Read the model definition and answer for the solid it produces. Units are mm, in the model's axes. Face numbers are marked on the shaded views. A direction names the side the tool comes from. Round coordinates to 2 decimals unless told otherwise and drop trailing zeros. Order: outer loops, then holes, each group sorted by start corner. A loop starts at its lowest first (then second) coordinate and runs counter-clockwise, first axis right, second up. Notation, with made-up numbers: (72, 40) - (84, 40) arc R17 ccw to (84, 70) - close; hole circle Ø10 at (37, -31). An arc over 180 degrees is marked (long way). Put each result on its own line as item: value. Start each with the question number.
Q1. Section D-D on y = -120 is taken. Give the vertices of the cut face in (x, z).
Q2. Section C-C on z = 0 is taken. Give the vertices of the cut face in (x, y).
Q3. Which of the six approach directions +Z, -Z, +X, -X, +Y, -Y give full straight-line access (tool end or side, diameter ignored) to the marked faces 5, 6 and 7?
Q4. Find the intervals of material crossed by line 1 along Y through (x, z) = (0, -2.25); line 2 along Y through (x, z) = (3.5, -7.25); line 3 along Y through (x, z) = (-1, 1.5), in increasing order. Write a range as from..to.
Q5. Each of these flat-tipped pins is pushed along its axis until it touches: pin 1 Ø2 at (x, y) = (10, -40) entering from -Z; pin 2 Ø12 at (x, y) = (-3, -66.5) entering from +Z; pin 3 Ø6 at (y, z) = (-37.5, 0.5) entering from -X; pin 4 Ø5.5 at (x, y) = (2.5, 21) entering from +Z. Where does it stop, or does it pass through?
Q6. Section B-B on x = 0 is taken. Give the vertices of the cut face in (y, z), then the cut area to 3 significant figures.
Q7. Section A-A on y = 0 is taken. Give the vertices of the cut face in (x, z), then the cut area to 3 significant figures.
Q8. For a pull along Y with two mould halves and no side action, classify the marked faces 1, 2, 3 and 4 as pulls with the +Y half, pulls with the -Y half, needs draft (parallel to the pull), parting line crosses it, or undercut.
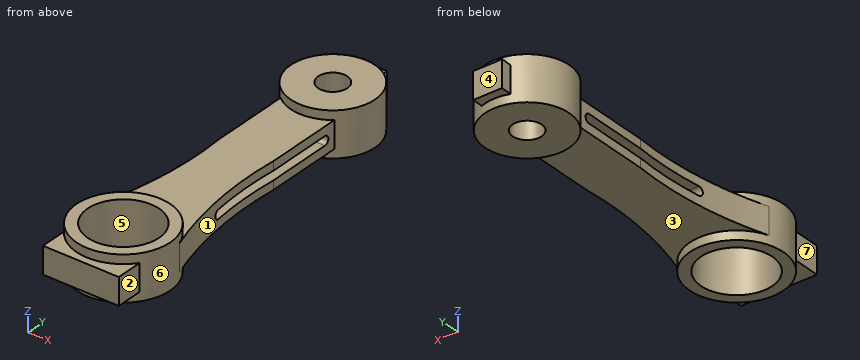
from build123d import *

# Parameters (mm, degrees)
IZIM2_R                       = 18.879465786
IZIM2_R_2                     = 6.5
Y_KSEKLIK_EKSTR_ZYON1_DEPTH   = 10
IZIM2_R_3                     = 21
IZIM2_R_4                     = 16
Y_KSEKLIK_EKSTR_ZYON1_2_DEPTH = 10
Y_KSEKLIK_EKSTR_ZYON3_DEPTH   = 6
Y_KSEKLIK_EKSTR_ZYON4_DEPTH   = 6
KES_EKSTR_ZYON1_START         = 6
KES_EKSTR_ZYON1_DEPTH         = 16


with BuildPart() as part:
    # izim2 → Y_kseklik-Ekstr_zyon1 (new body, symmetric)
    with BuildSketch(Plane.XY):
        Circle(IZIM2_R)
        Circle(IZIM2_R_2, mode=Mode.SUBTRACT)
    extrude(amount=Y_KSEKLIK_EKSTR_ZYON1_DEPTH, both=True)



with BuildPart() as body_2:
    # izim2 → Y_kseklik-Ekstr_zyon1 2 (new body, symmetric)
    with BuildSketch(Plane.XY):
        with Locations((0, -120)):
            Circle(IZIM2_R_3)
        with Locations((0, -120)):
            Circle(IZIM2_R_4, mode=Mode.SUBTRACT)
    extrude(amount=Y_KSEKLIK_EKSTR_ZYON1_2_DEPTH, both=True)


with BuildPart() as part_1:
    add(part.part)

    add(body_2.part)  # Y_kseklik-Ekstr_zyon3 merges body 2
    # izim2_8 → Y_kseklik-Ekstr_zyon3 (add, symmetric)
    with BuildSketch(Plane.XY):
        with BuildLine():
            ThreePointArc((12.082858103, -14.506507796), (0, -18.879465786), (-12.082858103, -14.506507796))
            Line((-12.082858103, -14.506507796), (-12.082858103, -49.506507796))
            ThreePointArc((-12.082858103, -49.506507796), (-12.752926263, -81.777932893), (-19.888250818, -113.257783792))
            ThreePointArc((-19.888250818, -113.257783792), (0, -99), (19.888250818, -113.257783792))
            ThreePointArc((19.888250818, -113.257783792), (12.752926263, -81.777932893), (12.082858103, -49.506507796))
            Line((12.082858103, -49.506507796), (12.082858103, -14.506507796))
        make_face()
    extrude(amount=Y_KSEKLIK_EKSTR_ZYON3_DEPTH, both=True)

    # izim2_9 → Y_kseklik-Ekstr_zyon4 (add, symmetric)
    with BuildSketch(Plane.XY):
        with BuildLine():
            Line((-6.5, 22.725242689), (-6.5, 17.725242689))
            ThreePointArc((-6.5, 17.725242689), (0, 18.879465786), (6.5, 17.725242689))
            Line((6.5, 17.725242689), (6.5, 22.725242689))
            Line((6.5, 22.725242689), (-6.5, 22.725242689))
        make_face()
        with BuildLine():
            ThreePointArc((17, -132.328828006), (0, -141), (-17, -132.328828006))
            Line((-17, -132.328828006), (-17, -144.328828006))
            Line((-17, -144.328828006), (17, -144.328828006))
            Line((17, -144.328828006), (17, -132.328828006))
        make_face()
    extrude(amount=Y_KSEKLIK_EKSTR_ZYON4_DEPTH, both=True)

    # izim4 → Kes-Ekstr_zyon1 (cut, through all)
    with BuildSketch(Plane(origin=(0, 0, 0), x_dir=(0, 0, -1), z_dir=(1, 0, 0)).offset(KES_EKSTR_ZYON1_START)):
        with BuildLine():
            Line((2, -20), (2, -82))
            ThreePointArc((2, -82), (0, -84), (-2, -82))
            Line((-2, -82), (-2, -20))
            ThreePointArc((-2, -20), (0, -18), (2, -20))
        make_face()
    kes_ekstr_zyon1 = extrude(amount=KES_EKSTR_ZYON1_DEPTH, mode=Mode.SUBTRACT)

    # Aynalama1: Kes-Ekstr_zyon1 across plane
    add(kes_ekstr_zyon1.mirror(Plane(origin=(0, 0, 0), x_dir=(0, 0, 1), z_dir=(1, 0, 0))), mode=Mode.SUBTRACT)


solid = part_1.part
Findings:
1. outline: (-21, -10) - (-16, -10) - (-16, 10) - (-21, 10) - close; (16, -10) - (21, -10) - (21, 10) - (16, 10) - close
2. outline: (-19.89, -113.26) arc R21 ccw to (-17, -132.33) - (-17, -144.33) - (17, -144.33) - (17, -132.33) arc R21 ccw to (19.89, -113.26) arc R159.96 cw to (13.04, -84) - (6, -84) - (6, -18) - (12.08, -18) - (12.08, -14.51) arc R18.88 ccw to (6.5, 17.73) - (6.5, 22.73) - (-6.5, 22.73) - (-6.5, 17.73) arc R18.88 ccw to (-12.08, -14.51) - (-12.08, -18) - (-6, -18) - (-6, -84) - (-13.04, -84) arc R159.96 cw to start; hole circle Ø32 at (0, -120); hole circle Ø13 at (0, 0)
3. face 5: +Z, -Z
3. face 6: none
3. face 7: +Z, -Z, -X, -Y
4. line 1: -144.33..-136, -104..-6.5, 6.5..22.73
4. line 2: -140.71..-135.61, -104.39..-99.29, -18.55..-5.48, 5.48..18.55
4. line 3: -144.33..-135.97, -104.03..-6.42, 6.42..22.73
5. pin 1: z = -6
5. pin 2: z = 6
5. pin 3: x = -12.08
5. pin 4: z = 10
6. outline: (-144.33, -6) - (-141, -6) - (-141, -10) - (-136, -10) - (-136, 10) - (-141, 10) - (-141, 6) - (-144.33, 6) - close; (-104, -10) - (-99, -10) - (-99, -6) - (-18.88, -6) - (-18.88, -10) - (-6.5, -10) - (-6.5, 10) - (-18.88, 10) - (-18.88, 6) - (-99, 6) - (-99, 10) - (-104, 10) - close; (6.5, -10) - (18.88, -10) - (18.88, -6) - (22.73, -6) - (22.73, 6) - (18.88, 6) - (18.88, 10) - (6.5, 10) - close
6. area: 1,740 mm2
7. outline: (-18.88, -10) - (-6.5, -10) - (-6.5, 10) - (-18.88, 10) - close; (6.5, -10) - (18.88, -10) - (18.88, 10) - (6.5, 10) - close
7. area: 495 mm2
8. face 1: undercut
8. face 2: needs draft
8. face 3: undercut
8. face 4: pulls with the +Y half
